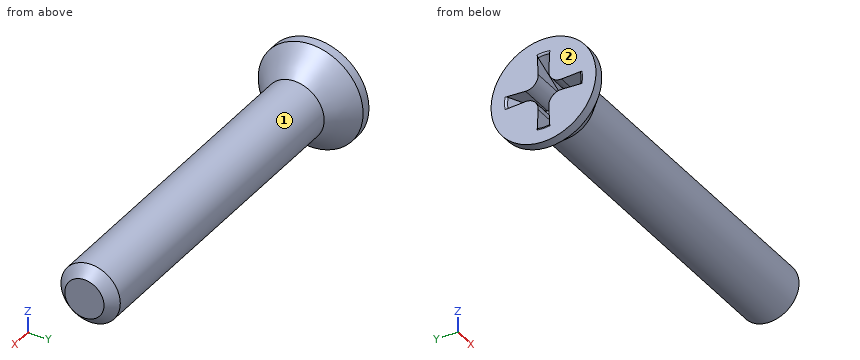
Autodesk Inventor part; units mm, degrees
ref_plane "Work Plane2" through (2.032, 0, 0) normal (0, 1, 0) x (1, 0, 0)
ref_plane "YZ Plane" through (0, 0, 0) normal (1, 0, 0) x (0, 1, 0)
ref_plane "XZ Plane" through (0, 0, 0) normal (0, 1, 0) x (-1, 0, 0)
sketch "Sketch1" plane through (0, 0, 0) normal (0, 0, 1) x (1, 0, 0)
  line L0 (2.6924, 0) -> (22.225, 0)
  line L1 (22.225, 0) -> (22.225, 1.7526)
  line L2 (22.225, 1.7526) -> (2.1082, 1.7526)
  line L3 (0.5596, 3.0988) -> (0, 3.0988)
  line L4 (-4.445, 0) -> (26.67, 0)
  line L5 (0, -0.6198) -> (0, 3.7186)
  line L6 (0, 2.2098) -> (2.0648, 1.1803)
  line L7 (2.0648, 1.1803) -> (2.6924, 0)
  line L8 (2.1082, 1.7526) -> (0.5596, 3.0988)
  line L9 (0, 3.0988) -> (0, 2.2098)
  dimension "d2" = 3.5052
  dimension "d3" = 6.1976
  dimension "d4" = 2.6924
  dimension "d5" = 4.4196
  dimension "d6" = 26.5
  dimension "d7" = 62
  dimension "d13" = 41
  dimension "d14" = 2.1082
  dimension "d15" = 22.225
revolve "Body" add sketch "Sketch1" angle 360 about axis through (2.6924, 0, 0) along (1, 0, 0) contours L7 L6 L5 L3 L8 L2 L1 L0
sketch "Sketch2" plane through (0, 0, 0) normal (-1, 0, 0) x (0, 0, 1)
  line L0 (0, -4.3383) -> (0, 4.3383)
  line L1 (-4.3383, 0) -> (4.3383, 0)
  line L2 (0, 2.2098) -> (0, 0) construction
  line L3 (0, 0) -> (2.2098, 0) construction
  arc A0 (0.7366, 0) -> (0, 0.7366) centre (0, 0) ccw
  line L4 (0, 0) -> (0.7947, 0.7947) construction
  arc A1 (1.1049, 0) -> (0, 1.1049) centre (0, 0) ccw construction
  line L5 (0.3683, 2.1789) -> (0.3131, 1.0596)
  line L6 (2.1789, 0.3683) -> (1.0596, 0.3131)
  arc A2 (0.3131, 1.0596) -> (1.0596, 0.3131) centre (1.0245, 1.0245) ccw
  arc A3 (2.2098, 0) -> (2.1789, 0.3683) centre (0, 0) ccw
  arc A4 (0.3683, 2.1789) -> (0, 2.2098) centre (0, 0) ccw
  arc A5 (2.1789, 0.3683) -> (0.3683, 2.1789) centre (0, 0) ccw
  line L7 (0.3683, -2.1789) -> (0.3131, -1.0596)
  line L8 (2.1789, -0.3683) -> (1.0596, -0.3131)
  arc A6 (1.0596, -0.3131) -> (0.3131, -1.0596) centre (1.0245, -1.0245) ccw
  arc A7 (2.1789, -0.3683) -> (2.2098, 0) centre (0, 0) ccw
  arc A8 (0, -2.2098) -> (0.3683, -2.1789) centre (0, 0) ccw
  arc A9 (0.3683, -2.1789) -> (2.1789, -0.3683) centre (0, 0) ccw
  line L9 (-0.3683, 2.1789) -> (-0.3131, 1.0596)
  line L10 (-2.1789, 0.3683) -> (-1.0596, 0.3131)
  arc A10 (-1.0596, 0.3131) -> (-0.3131, 1.0596) centre (-1.0245, 1.0245) ccw
  arc A11 (-2.1789, 0.3683) -> (-2.2098, 0) centre (0, 0) ccw
  arc A12 (0, 2.2098) -> (-0.3683, 2.1789) centre (0, 0) ccw
  arc A13 (-0.3683, 2.1789) -> (-2.1789, 0.3683) centre (0, 0) ccw
  arc A14 (-2.1789, -0.3683) -> (-0.3683, -2.1789) centre (0, 0) ccw
  arc A15 (-0.3683, -2.1789) -> (0, -2.2098) centre (0, 0) ccw
  arc A16 (-2.2098, 0) -> (-2.1789, -0.3683) centre (0, 0) ccw
  line L11 (-2.1789, -0.3683) -> (-1.0596, -0.3131)
  arc A17 (-0.3131, -1.0596) -> (-1.0596, -0.3131) centre (-1.0245, -1.0245) ccw
  line L12 (-0.3683, -2.1789) -> (-0.3131, -1.0596)
  dimension "d18" = 45
  dimension "d19" = 1.4732
  dimension "d20" = 2.2098
  dimension "d21" = 4.4196
  dimension "d22" = 0.3683
extrude "Slot" add sketch "Sketch2" against normal up to next contours A2 L5 A5 L6 | L9 A10 L10 A13 | L7 A6 L8 A9 | A14 L11 A17 L12
fillet "Fillet1" radius 0.1473 4 edges at (0, 2.2098, 0) (0, 0, 2.2098) (0, -2.2098, 0) (0, 0, -2.2098)
thread "Thread"
chamfer "Chamfer1" distance 0.5953 distance2 0.5953 1 edges at (22.225, -1.7526, 0) measured on face at (22.225, -0.5173, -0.2715)
ref_plane "Work Plane2" through (2.032, 0, 0) normal (0, 1, 0) x (1, 0, 0)
equation "\"d2\" = GD"
equation "\"d3\" = KOD"
equation "\"d4\" = INTI"
equation "\"d5\" = SDM"
equation "\"d13\" = 0.5 * SEWI"
equation "\"d14\" = KOH"
equation "\"d15\" = NLG"
equation "\"d19\" = 0.333333 * SDM"
equation "\"d20\" = 0.5 * SDM"
equation "\"d21\" = SDM"
equation "\"d22\" = 0.5 * SBR"
equation "\"d45\" = INTI"
equation "\"d25\" = 0.2 * SBR"
equation "\"d9\" = GEL"
equation "\"d11\" = -0.5 * SPD + 0.5 * GD"
equation "\"d12\" = GUL"
equation "\"GD\" = NND"
equation "\"NLG\" = 22.225"
equation "\"GEL\" = 18.13243"
equation "\"KOD\" = 6.1976"
equation "\"KOH\" = 2.1082"
equation "\"SDM\" = 4.4196"
equation "\"INTI\" = 2.6924"
equation "\"SBR\" = 0.7366"
equation "\"GUL\" = 0.75 * GAL"
equation "\"SPD\" = 2.31458"
equation "\"SEWI\" = 82deg"
equation "\"d0\" = NLG"
equation "\"d1\" = KOH"
equation "\"d17\" = SDM"
equation "\"TOA\" = 30deg"
equation "\"THREADDIA\" = 3.5052"
equation "\"BDM\" = NND"
equation "\"NND\" = 3.5052"
equation "\"GAL\" = 0.79375"
equation "\"GD1\" = SPD"
properties part number "ANSI B18.6.3 - 6-32 x 7/8, CRFCHMSTII(5)" material "Steel, Mild"
For this review, take the finished solid that the model builds, in its own axes (mm). Face numbers are marked on the shaded views. A direction names the side the tool comes from. Round coordinates to 2 decimals unless told otherwise and drop trailing zeros. Loops run counter-clockwise (first coordinate to the right, second up) from the corner with the lowest first, then second, coordinate; pieces in that order, holes last.
Q1. Insertion check: pin 1 Ø1 at (x, y) = (8.5, -0.5) entering from +Z; pin 2 Ø1 at (x, z) = (12.5, 1.5) entering from +Y. Each pin has a flat end and moves straight along its axis. Give the tip position at first contact, or say it passes through.
Result sheet:
pin 1: stops at z = 1.75
pin 2: stops at y = 1.44
Q2. Add section A-A on x = 4.25. Write out the cut boundary in (y, z), plus the area to 3 significant figures.
Result sheet:
outline: circle Ø3.51 at (0, 0)
area: 9.65 mm2
Q3. Machinability: for the marked faces 1 and 2, which of the approach directions +Z, -Z, +X, -X, +Y, -Y give a long, thin tool a straight path to every point of the face, cutting with its end or side? Answer none if there is none.
Result sheet:
face 1: +X
face 2: +Z, -Z, -X, +Y, -Y
Q4. To check wall thickness, follow line 1 along Z through (x, y) = (6.5, 0); line 2 along Z through (x, y) = (1.25, 1.5); line 3 along Z through (x, y) = (12.75, 1.5). State the ranges of each line that lie inside material, in increasing order.
Result sheet:
line 1: z = -1.75 to 1.75
line 2: z = -2 to -0.33, 0.33 to 2
line 3: z = -0.91 to 0.91
